Verification items for the finished model (mm, model axes). Give positions to 0.01 mm unless a question says otherwise; leave off trailing zeros. Order: outer loops, then holes, each group sorted by start corner. A loop starts at its lowest first (then second) coordinate and runs counter-clockwise, first axis right, second up. Notation, with made-up numbers: (-11.5, 27) - (36.5, 27) arc R23 ccw to (36.5, 46) - close; hole circle Ø4 at (-32, 59.5). An arc over 180 degrees is marked (long way). Answer as a JSON object with one key per item and string values.
```python
from build123d import *

# Parameters (mm, degrees)
SKETCH1_R           = 10
SKETCH1_R_2         = 1.778
BOSS_EXTRUDE1_DEPTH = 3


with BuildPart() as part:
    # Sketch1 → Boss-Extrude1 (new body)
    with BuildSketch(Plane(origin=(0, 0, 0), x_dir=(1, 0, 0), z_dir=(0, 1, 0))):
        Polygon((-250, -300), (-250, 400), (-150, 400), (-150, 500), (150, 500), (150, 400), (250, 400), (250, -300), (175, -300), (175, -500), (-175, -500), (-175, -300), align=None)
        with Locations(Location((133.9, -400, 0), (0, 0, 270))):
            Circle(SKETCH1_R, mode=Mode.SUBTRACT)
        with Locations(Location((-133.9, -400, 0), (0, 0, 90))):
            Circle(SKETCH1_R, mode=Mode.SUBTRACT)
        with Locations(Location((140, 466.9494, 0), (0, 0, 270))):
            Circle(SKETCH1_R_2, mode=Mode.SUBTRACT)
        with Locations(Location((140, 440, 0), (0, 0, 270))):
            Circle(SKETCH1_R_2, mode=Mode.SUBTRACT)
        with Locations(Location((-140, 466.9494, 0), (0, 0, 90))):
            Circle(SKETCH1_R_2, mode=Mode.SUBTRACT)
        with Locations(Location((-140, 440, 0), (0, 0, 90))):
            Circle(SKETCH1_R_2, mode=Mode.SUBTRACT)
    extrude(amount=BOSS_EXTRUDE1_DEPTH)


solid = part.part
```
(1) Release check for a two-part mould opening along X. For faces 1 (the flat face through (3, 0, -7)), 2 (the cylindrical face through (124.14, 1.48, 397.83)) record: pulls with the +X half, pulls with the -X half, needs draft (parallel to the pull), parting line crosses it, or undercut.
Computed values:
{"face 1": "needs draft", "face 2": "undercut"}
(2) Gauge pin test, flat ends, axial feed: pin 1 Ø1.5 at (x, y) = (206.5, 1) entering from +Z; pin 2 Ø1.5 at (x, y) = (187, 1) entering from -Z; pin 3 Ø0.9 at (y, z) = (2, -450) entering from +X. Record the tip position at first contact, or that the pin passes through.
Computed values:
{"pin 1": "stops at z = 300", "pin 2": "stops at z = -400", "pin 3": "stops at x = 150"}
(3) Material ranges on line 1 along X through (y, z) = (0.85, -440); line 2 along Z through (x, y) = (-133, 0.15); line 3 along X through (y, z) = (1.9, 400), recorded low to high. Write a range as [from, to].
Computed values:
{"line 1": "x = [-150, -141.78], [-138.22, 138.22], [141.78, 150]", "line 2": "z = [-500, 390.04], [409.96, 500]", "line 3": "x = [-175, -143.9], [-123.9, 123.9], [143.9, 175]"}
(4) Section check B-B (y = 1.45). Record the cut outline in (x, z), then the cut area to 3 significant figures.
Computed values:
{"outline": "(-250, -400) - (-150, -400) - (-150, -500) - (150, -500) - (150, -400) - (250, -400) - (250, 300) - (175, 300) - (175, 500) - (-175, 500) - (-175, 300) - (-250, 300) - close; hole circle Ø20 at (-133.9, 400); hole circle Ø3.56 at (-140, -466.95); hole circle Ø3.56 at (-140, -440); hole circle Ø20 at (133.9, 400); hole circle Ø3.56 at (140, -466.95); hole circle Ø3.56 at (140, -440)", "area": "449,000 mm²"}
(5) Section check A-A (z = 400). Record the cut outline in (x, y).
Computed values:
{"outline": "(-175, 0) - (-143.9, 0) - (-143.9, 3) - (-175, 3) - close; (-123.9, 0) - (123.9, 0) - (123.9, 3) - (-123.9, 3) - close; (143.9, 0) - (175, 0) - (175, 3) - (143.9, 3) - close"}
